The model under review builds one solid part; all positions refer to its coordinate system, in mm. A direction names the side the tool comes from. Coordinates: 2 decimals unless noted, no trailing zeros. Write each loop counter-clockwise with the first axis right and the second up, starting at its lowest first coordinate (ties: lowest second). Pieces come first, ordered by that corner, then holes. Notation, with made-up numbers: (-3, -3) -> (26, -3) arc R26 ccw to (26, 22) -> close; hole circle Ø5 at (36.25, 47). An arc over 180 degrees is marked (long way). Write each question's results on one line, items separated by ' | '.
Autodesk Inventor part; units mm, degrees
ref_plane "YZ Plane" through (0, 0, 0) normal (1, 0, 0) x (0, 1, 0)
ref_plane "XZ Plane" through (0, 0, 0) normal (0, 1, 0) x (-1, 0, 0)
ref_plane "XY Plane" through (0, 0, 0) normal (0, 0, 1) x (1, 0, 0)
sketch "Sketch1" plane through (0, 0, 0) normal (0, 1, 0) x (-1, 0, 0)
  circle A0 centre (7.5, 0) radius 13
  line L0 (-17.5, 45) -> (32.5, 45)
  line L1 (32.5, 45) -> (32.5, 0)
  line L2 (-17.5, 45) -> (-17.5, 0)
  arc A1 (-17.5, 0) -> (32.5, 0) centre (7.5, 0) ccw
  point P0 (0, 0)
  dimension "d1" = 26
  dimension "d6" = 50
  dimension "d29" = 45
extrude "Base" add sketch "Sketch1" along normal blind 34
sketch "Sketch3" plane through (0, 34, 0) normal (0, 1, 0) x (1, 0, 0)
  circle A0 centre (-7.5, 0) radius 13
  line L0 (-7.5, 0) -> (-25, 0)
  line L1 (-25, 0) -> (10, 0)
  circle A1 centre (-25, 0) radius 2.6035
  point P0 (0, 0)
  dimension "d10" = 35
  dimension "d11" = 5.207
extrude "Screw Hole" cut sketch "Sketch3" against normal through all contours A1
pattern_circular "Circular Pattern1" count 4 over 360 about axis through (-7.5, 0, 0) along (0, 1, 0) of "Screw Hole"
sketch "Sketch4" plane through (-32.5, 0, 45) normal (0, 0, 1) x (1, 0, 0)
  line L0 (0, 0) -> (0, 34)
  line L1 (0, 17) -> (50, 17)
  line L2 (50, 0) -> (50, 34)
  line L3 (25, 17) -> (25, 25.625)
  line L4 (25, 25.625) -> (33.5, 25.625)
  circle A0 centre (33.5, 25.625) radius 2.6035
  point P0 (32.5, 0)
  dimension "d17" = 8.625
  dimension "d18" = 8.5
  dimension "d19" = 5.207
extrude "Mount Holes" cut sketch "Sketch4" against normal blind 20
pattern_linear "Rectangular Pattern1" count 2 spacing 17 along (0, -1, 0) count 2 spacing 17.25 along (-1, 0, 0) of "Mount Holes"
properties part number "LimbAttachment"
Q1. Clearance check with flat-ended pins moving along their axes: P1, Ø5, axis at x = -9, y = 23.5, coming from the -Z side; P2, Ø2, axis at y = 17.5, z = -13.5, coming from the +X side; P3, Ø3, axis at y = 30, z = -5.5, coming from the -X side. State where each tip first meets the part, or that it passes through.
Solution:
P1: z = -25 | P2: x = 14.15 | P3: x = -32.18
Q2. Draft analysis for pull direction X (two halves, no side actions). For faces 3 (the flat face through (-7, 17, 45)), 4 (the flat face through (17.5, 17, 23)), 5 (the flat face through (-16, 9, 25)), 6 (the cylindrical face through (0.661, 28.206, 35.14)), state which applies: pulls with the +X half, pulls with the -X half, needs draft (parallel to the pull), parting line crosses it, or undercut.
Solution:
face 3: needs draft | face 4: pulls with the +X half | face 5: undercut | face 6: undercut
Q3. Add section B-B (y = 16). Write out the cut boundary in (x, z).
Solution:
outline: (-32.5, 0) arc R25 ccw to (17.5, 0) -> (17.5, 45) -> (-32.5, 45) -> close; hole circle Ø5.21 at (-25, 0); hole circle Ø26 at (-7.5, 0); hole circle Ø5.21 at (-7.5, -17.5); hole circle Ø5.21 at (-7.5, 17.5); hole circle Ø5.21 at (10, 0)
Q4. Add section A-A (x = -7.5). Write out the cut boundary in (y, z), plus the area to 3 significant figures.
Solution:
outline: (0, -25) -> (34, -25) -> (34, -20.1) -> (0, -20.1) -> close; (0, -14.9) -> (34, -14.9) -> (34, -13) -> (0, -13) -> close; (0, 13) -> (34, 13) -> (34, 14.9) -> (0, 14.9) -> close; (0, 20.1) -> (34, 20.1) -> (34, 45) -> (0, 45) -> close | area: 1,140 mm²
Q5. Add section D-D (z = -7). Write out the cut boundary in (x, y), plus the area to 3 significant figures.
Solution:
outline: (-31.5, 0) -> (-18.45, 0) -> (-18.45, 34) -> (-31.5, 34) -> close; (3.45, 0) -> (16.5, 0) -> (16.5, 34) -> (3.45, 34) -> close | area: 887 mm²
Q6. For line 1 (Y direction, x = -16, z = 39.5); line 2 (Z direction, x = -7, y = 20) (3 decimals); line 3 (X direction, y = 8.5, z = 28), list the stretches that pass through material, from the lowest coordinate up. Write a range as from..to.
Solution:
line 1: 0..6.03, 11.22..23.03, 28.22..34 | line 2: -24.995..-20.055, -14.945..-12.99, 12.99..14.945, 20.055..45 | line 3: -32.5..-18.85, -13.65..-1.6, 3.6..17.5
Q7. Machinability: for faces 1 (the flat face through (-32.5, 17, 23)), 2 (the flat face through (-16, 26, 25)), which of the approach directions +Z, -Z, +X, -X, +Y, -Y give a long, thin tool a straight path to every point of the face, cutting with its end or side? Answer none if there is none.
Solution:
face 1: +Z, -Z, -X, +Y, -Y | face 2: +Z
Q8. Add section C-C (x = -25). Write out the cut boundary in (y, z), plus the area to 3 significant figures.
Solution:
outline: (0, -17.85) -> (34, -17.85) -> (34, -2.6) -> (0, -2.6) -> close; (0, 2.6) -> (34, 2.6) -> (34, 45) -> (0, 45) -> close | area: 1,960 mm²
